Could you check a few things on this model? Use its own coordinates, in mm. A direction names the side the tool comes from. Round coordinates to 2 decimals unless told otherwise and drop trailing zeros. Loops run counter-clockwise (first coordinate to the right, second up) from the corner with the lowest first, then second, coordinate; pieces in that order, holes last. Notation, with made-up numbers: (44.25, -24.75) -> (87.25, -24.75) arc R15 ccw to (87.25, -1.75) -> close; hole circle Ø2 at (33.25, 61). An arc over 180 degrees is marked (long way). Write each question's results on one line, items separated by ' | '. Start each with the question number.
1) For P1, Ø1.9, axis at x = -18, y = -2.5, coming from the +Z side; P2, Ø5, axis at x = 1.5, y = -4.5, coming from the +Z side; P3, Ø3, axis at x = 6, y = -8.5, coming from the -Z side, each with a flat end and sliding along its axis, tell me the tip position at first contact or that it passes through.
2) Imagine slicing it at B-B, the plane y = -10.5. Give the number of separate pieces and of enclosed holes in the cut face, plus the area to 3 significant figures.
3) If I drill on probe 1 along X at (y, z) = (-8, -3.5); probe 2 along X at (y, z) = (-2.75, 13.5); probe 3 along Z at (x, y) = (9.5, -3.75), over which ranges is the centre line in solid material (lowest first)?
4) Imagine slicing it at C-C, the plane z = 19. List the corners of the cut face in (x, y) for me.
5) Which directions (+Z, -Z, +X, -X, +Y, -Y) give clear straight access to the entire face, cutting with the end or side of a thin tool? Please do faces 1 (the flat face through (-18, -7.618, 9)), 2 (the flat face through (33.845, -10, 9)), 3 (the cylindrical face through (28.931, -3.131, 19.673)), 4 (the flat face through (16, 0, -2)), 5 (the cylindrical face through (9.069, -5.649, 52.504)).
6) Imagine slicing it at A-A, the plane x = -4. List the corners of the cut face in (y, z) for me, plus the area to 3 significant figures.
from build123d import *

# Parameters (mm, degrees)
F0_W      = 57.4675095904
F0_H      = 88.5825127872
F1_DEPTH  = 12.7
F3_DEPTH  = 57.4685095904
F4_W      = 50.3555086569
F4_H      = 81.4705118537
F5_DEPTH  = 6.35
F6_R      = 0.7619995332
F8_DEPTH  = 6.35
F11_DEPTH = 56.388
F12_DEPTH = 1.0668
F15_DEPTH = 6.35
F16_DEPTH = 3.81


# Not quite as in the source:
# - a feature of the source that left no trace in its solid (it failed there, or was rolled back) is left out


with BuildPart() as f1:
    # F0 (on Front) → F1 (new body)
    with BuildSketch(Plane.XZ):
        with Locations((8.6671997911, 9.8971910775)):
            Rectangle(F0_W, F0_H)
        with BuildLine():
            ThreePointArc((-13.7333380541, -11.5169252571), (-11.8734661146, -7.0267971965), (-7.3833380541, -5.1669252571))
            Line((-7.3833380541, -5.1669252571), (24.6841715364, -5.1669252571))
            ThreePointArc((24.6841715364, -5.1669252571), (29.1742995969, -7.0267971965), (31.0341715364, -11.5169252571))
            Line((31.0341715364, -11.5169252571), (31.0341715364, -21.9464536455))
            ThreePointArc((31.0341715364, -21.9464536455), (29.1742995969, -26.436581706), (24.6841715364, -28.2964536455))
            Line((24.6841715364, -28.2964536455), (-7.3833380541, -28.2964536455))
            ThreePointArc((-7.3833380541, -28.2964536455), (-11.8734661146, -26.436581706), (-13.7333380541, -21.9464536455))
            Line((-13.7333380541, -21.9464536455), (-13.7333380541, -11.5169252571))
        make_face(mode=Mode.SUBTRACT)
        with BuildLine():
            ThreePointArc((-13.9270129099, 15.1340997942), (-12.0671409704, 19.6242278547), (-7.5770129099, 21.4840997942))
            Line((-7.5770129099, 21.4840997942), (24.4904966805, 21.4840997942))
            ThreePointArc((24.4904966805, 21.4840997942), (28.980624741, 19.6242278547), (30.8404966805, 15.1340997942))
            Line((30.8404966805, 15.1340997942), (30.8404966805, 4.7045714058))
            ThreePointArc((30.8404966805, 4.7045714058), (28.980624741, 0.2144433453), (24.4904966805, -1.6454285942))
            Line((24.4904966805, -1.6454285942), (-7.5770129099, -1.6454285942))
            ThreePointArc((-7.5770129099, -1.6454285942), (-12.0671409704, 0.2144433453), (-13.9270129099, 4.7045714058))
            Line((-13.9270129099, 4.7045714058), (-13.9270129099, 15.1340997942))
        make_face(mode=Mode.SUBTRACT)
        with BuildLine():
            ThreePointArc((-13.7165550041, 42.8851837456), (-11.8566830647, 47.3753118062), (-7.3665550041, 49.2351837456))
            Line((-7.3665550041, 49.2351837456), (24.7009545863, 49.2351837456))
            ThreePointArc((24.7009545863, 49.2351837456), (29.1910826468, 47.3753118062), (31.0509545863, 42.8851837456))
            Line((31.0509545863, 42.8851837456), (31.0509545863, 32.4556553572))
            ThreePointArc((31.0509545863, 32.4556553572), (29.1910826468, 27.9655272967), (24.7009545863, 26.1056553572))
            Line((24.7009545863, 26.1056553572), (-7.3665550041, 26.1056553572))
            ThreePointArc((-7.3665550041, 26.1056553572), (-11.8566830647, 27.9655272967), (-13.7165550041, 32.4556553572))
            Line((-13.7165550041, 32.4556553572), (-13.7165550041, 42.8851837456))
        make_face(mode=Mode.SUBTRACT)
    extrude(amount=F1_DEPTH)

    # F2 (on face) → F3 (cut, through all)
    with BuildSketch(Plane.YZ.offset(37.4009545863)):
        with BuildLine():
            ThreePointArc((-12.7, 54.1884474711), (-5.5566722855, 52.456369837), (0, 47.6448610425))
            Line((0, 47.6448610425), (0, 54.1884474711))
            Line((0, 54.1884474711), (-12.7, 54.1884474711))
        make_face()
    extrude(amount=-F3_DEPTH, mode=Mode.SUBTRACT)

    # F4 (on face) → F5 (cut)
    with BuildSketch(Plane.XZ.offset(12.7)):
        with Locations((8.6671997911, 9.8971910775)):
            Rectangle(F4_W, F4_H)
        with BuildLine():
            Line((-13.7333380541, -21.9464536455), (-13.7333380541, -11.5169252571))
            ThreePointArc((-13.7333380541, -11.5169252571), (-11.8734661146, -7.0267971965), (-7.3833380541, -5.1669252571))
            Line((-7.3833380541, -5.1669252571), (24.6841715364, -5.1669252571))
            ThreePointArc((24.6841715364, -5.1669252571), (29.1742995969, -7.0267971965), (31.0341715364, -11.5169252571))
            Line((31.0341715364, -11.5169252571), (31.0341715364, -21.9464536455))
            ThreePointArc((31.0341715364, -21.9464536455), (29.1742995969, -26.436581706), (24.6841715364, -28.2964536455))
            Line((24.6841715364, -28.2964536455), (-7.3833380541, -28.2964536455))
            ThreePointArc((-7.3833380541, -28.2964536455), (-11.8734661146, -26.436581706), (-13.7333380541, -21.9464536455))
        make_face(mode=Mode.SUBTRACT)
        with BuildLine():
            Line((24.4904966805, -1.6454285942), (-7.5770129099, -1.6454285942))
            ThreePointArc((-7.5770129099, -1.6454285942), (-12.0671409704, 0.2144433453), (-13.9270129099, 4.7045714058))
            Line((-13.9270129099, 4.7045714058), (-13.9270129099, 15.1340997942))
            ThreePointArc((-13.9270129099, 15.1340997942), (-12.0671409704, 19.6242278547), (-7.5770129099, 21.4840997942))
            Line((-7.5770129099, 21.4840997942), (24.4904966805, 21.4840997942))
            ThreePointArc((24.4904966805, 21.4840997942), (28.980624741, 19.6242278547), (30.8404966805, 15.1340997942))
            Line((30.8404966805, 15.1340997942), (30.8404966805, 4.7045714058))
            ThreePointArc((30.8404966805, 4.7045714058), (28.980624741, 0.2144433453), (24.4904966805, -1.6454285942))
        make_face(mode=Mode.SUBTRACT)
        with BuildLine():
            ThreePointArc((-7.3665550041, 26.1056553572), (-11.8566830647, 27.9655272967), (-13.7165550041, 32.4556553572))
            Line((-13.7165550041, 32.4556553572), (-13.7165550041, 42.8851837456))
            ThreePointArc((-13.7165550041, 42.8851837456), (-11.8566830647, 47.3753118062), (-7.3665550041, 49.2351837456))
            Line((-7.3665550041, 49.2351837456), (24.7009545863, 49.2351837456))
            ThreePointArc((24.7009545863, 49.2351837456), (29.1910826468, 47.3753118062), (31.0509545863, 42.8851837456))
            Line((31.0509545863, 42.8851837456), (31.0509545863, 32.4556553572))
            ThreePointArc((31.0509545863, 32.4556553572), (29.1910826468, 27.9655272967), (24.7009545863, 26.1056553572))
            Line((24.7009545863, 26.1056553572), (-7.3665550041, 26.1056553572))
        make_face(mode=Mode.SUBTRACT)
    extrude(amount=-F5_DEPTH, mode=Mode.SUBTRACT)

    # F6 (on face) → F8 (join)
    with BuildSketch(Plane.XZ.offset(6.35)):
        with Locations((-14.4785545374, 48.6004470043)):
            Circle(F6_R)
        with Locations((31.8129541195, 48.6004470043)):
            Circle(F6_R)
    extrude(amount=F8_DEPTH)

    # F10 (on face) → F11 (join)
    with BuildSketch(Plane.YZ.offset(37.4009545863)):
        with BuildLine():
            Line((0, -34.3940653161), (-12.7, -34.3940653161))
            ThreePointArc((-12.7, -34.3940653161), (-6.35, -40.7440653161), (0, -34.3940653161))
        make_face()
    extrude(amount=-F11_DEPTH)

    # F12 (add): a face of the model
    f12_faces = [f1.faces().sort_by_distance(p)[0] for p in [
        (-18.9870454137, -6.35, -37.0890890192),
    ]]
    extrude(f12_faces, amount=F12_DEPTH)

    # F14 (on face) → F15 (cut)
    with BuildSketch(Plane(origin=(0, 0, 0), x_dir=(-1, 0, 0), z_dir=(0, 1, 0))):
        with BuildLine():
            Line((16.464073211, -26.9519573744), (16.464073211, -33.4652290945))
            ThreePointArc((16.464073211, -33.4652290945), (18.7668625115, -32.5113825349), (19.720709071, -30.2085932344))
            ThreePointArc((19.720709071, -30.2085932344), (18.7668625115, -27.9058039339), (16.464073211, -26.9519573744))
        make_face()
        with BuildLine():
            ThreePointArc((16.464073211, -26.9519573744), (13.2074373509, -30.2085932344), (16.464073211, -33.4652290945))
            Line((16.464073211, -33.4652290945), (16.464073211, -26.9519573744))
        make_face()
    extrude(amount=-F15_DEPTH, mode=Mode.SUBTRACT)

    # F13 (on face) → F16 (cut)
    with BuildSketch(Plane(origin=(-20.0665550041, 0, 0), x_dir=(0, -1, 0), z_dir=(-1, 0, 0))):
        with BuildLine():
            Line((0, -34.3940653161), (7.6183550991, -34.3940653161))
            Line((7.6183550991, -34.3940653161), (7.6183550991, 53.3373526242))
            ThreePointArc((7.6183550991, 53.3373526242), (3.3646993114, 51.0859593692), (0, 47.6448610425))
            Line((0, 47.6448610425), (0, -34.3940653161))
        make_face()
    extrude(amount=-F16_DEPTH, mode=Mode.SUBTRACT)


solid = f1.part
Checked values:
1) P1: z = -34.39 | P2: z = 53.11 | P3: z = -40.71
2) separate pieces: 3 | enclosed holes: 1 | area: 1,260 mm^2
3) probe 1: -20.07 to -16.51, 33.84 to 37.4 | probe 2: -16.26 to -13.93, 30.84 to 37.4 | probe 3: -40.19 to -28.3, -5.17 to -1.65, 21.48 to 26.11, 49.24 to 51.36
4) outline: (-20.07, -12.7) -> (-16.51, -12.7) -> (-16.51, -7.62) -> (-20.07, -7.62) -> close; (-16.26, -6.35) -> (-12.61, -6.35) -> (-12.61, 0) -> (-16.26, 0) -> close; (29.53, -6.35) -> (33.84, -6.35) -> (33.84, -12.7) -> (37.4, -12.7) -> (37.4, 0) -> (29.53, 0) -> close
5) face 1: +Z, -X, +Y | face 2: -Y | face 3: +Y, -Y | face 4: +Z, -Z, +X, -X, +Y | face 5: +Z, +X, -X, +Y
6) outline: (-12.7, -34.39) arc R6.35 ccw to (0, -34.39) -> (0, -28.3) -> (-6.35, -28.3) -> (-6.35, -30.84) -> (-12.7, -30.84) -> close; (-12.7, 50.63) -> (-6.35, 50.63) -> (-6.35, 49.24) -> (-1.3, 49.24) arc R15.6 ccw to (-12.7, 54.19) -> close; (-6.35, -5.17) -> (0, -5.17) -> (0, -1.65) -> (-6.35, -1.65) -> close; (-6.35, 21.48) -> (0, 21.48) -> (0, 26.11) -> (-6.35, 26.11) -> close | area: 207 mm^2
